from build123d import *

# Parameters (mm, degrees)
F0_R     = 33.274
F0_R_2   = 32.766
F1_DEPTH = 38.1
F2_R     = 33.274
F2_R_2   = 31.115
F3_DEPTH = 3.175


with BuildPart() as f1:
    # F0 (on Front) → F1 (new body)
    with BuildSketch(Plane.XZ):
        Circle(F0_R)
        Circle(F0_R_2, mode=Mode.SUBTRACT)
    extrude(amount=-F1_DEPTH)

    # F2 (on face) → F3 (join)
    with BuildSketch(Plane(origin=(0, 38.1, 0), x_dir=(-1, 0, 0), z_dir=(0, 1, 0))):
        Circle(F2_R)
        Circle(F2_R_2, mode=Mode.SUBTRACT)
    extrude(amount=F3_DEPTH)


solid = f1.part
Check sheet for the modelled part. Datum: model origin and axes. Units: mm. A direction names the side the tool comes from. Give positions to 0.01 mm unless a question says otherwise; leave off trailing zeros. Order: outer loops, then holes, each group sorted by start corner. A loop starts at its lowest first (then second) coordinate and runs counter-clockwise, first axis right, second up. Notation, with made-up numbers: M 39,66.25 L 45,66.25 A35 ccw 45,98.25 Z; hole C -31,38 d3. An arc over 180 degrees is marked long. Answer as CSV lines item,"result". Start each with the question number.
Item 1: Cross-section at A-A on x = 0. Enter the section's corners in (y, z) (3 decimals), plus the area to 3 significant figures.
Item 2: Tool access check on faces 3 (the face through (31.253, 18.783, 9.842)), 4 (the face through (-19.6, 41.275, -24.5)). Record the directions out of +Z, -Z, +X, -X, +Y, -Y that give a thin tool (end or side, any length) a straight path to the whole face; none if there is none.
Item 3: Mould release check, pull along Z, two halves, no side actions. Record for faces 1 (the face through (-29, 38.1, -12)), 2 (the face through (24.5, 0, -22)): +Z half, -Z half, draft (parallel to the pull), parting line (faces both ways), or undercut.
Item 4: Thickness scan on line 1 (Z direction, x = 0, y = 14.5); line 2 (Z direction, x = 15, y = 23.5); line 3 (X direction, y = 25, z = 6). Record the ranges inside material, lowest first. Write a range as [from, to].
Item 5: Cross-section at C-C on y = 23. Enter the section's corners in (x, z), plus the area to 3 significant figures.
Item 6: Cross-section at B-B on z = 0. Enter the section's corners in (x, y) (3 decimals).
Item 7: Gauge pin test, flat ends, axial feed: P1, Ø10, axis at x = -21, y = 23.5, coming from the -Z side; P2, Ø1.5, axis at x = 2.5, y = 15.5, coming from the +Z side; P3, Ø3, axis at y = 36, z = 25.5, coming from the +X side. Record the tip position at first contact, or that the pin passes through.
Established:
1,outline,"M 0,-33.274 L 41.275,-33.274 L 41.275,-31.115 L 38.1,-31.115 L 38.1,-32.766 L 0,-32.766 Z; M 0,32.766 L 38.1,32.766 L 38.1,31.115 L 41.275,31.115 L 41.275,33.274 L 0,33.274 Z"
1,area,"52.4 mm^2"
2,face 3,"-Y"
2,face 4,"+Z, -Z, +X, -X, +Y"
3,face 1,"undercut"
3,face 2,"draft"
4,line 1,"z = [-33.27, -32.77], [32.77, 33.27]"
4,line 2,"z = [-29.7, -29.13], [29.13, 29.7]"
4,line 3,"x = [-32.73, -32.21], [32.21, 32.73]"
5,outline,"C 0,0 d66.55; hole C 0,0 d65.53"
5,area,"105 mm^2"
6,outline,"M -33.274,0 L -32.766,0 L -32.766,38.1 L -31.115,38.1 L -31.115,41.275 L -33.274,41.275 Z; M 31.115,38.1 L 32.766,38.1 L 32.766,0 L 33.274,0 L 33.274,41.275 L 31.115,41.275 Z"
7,P1,"stops at z = -29.17"
7,P2,"stops at z = 33.23"
7,P3,"stops at x = 23.05"
